```python
from build123d import *

# Parameters (mm, degrees)
BASE_FLANGE1_DEPTH           = 3.175
SKETCH7_R                    = 2.15
CUT_EXTRUDE1_DEPTH           = 10
CUT_EXTRUDE2_DEPTH           = 10
SKETCHED_START               = 19.282254495
SKETCHED_BEND9_OUTLINE_W     = 16.753945323
SKETCHED_BEND9_OUTLINE_H     = 3.175
SKETCHED_BEND9_OUTLINE_W_2   = 24.844698194
SKETCHED_BEND9_OUTLINE_W_3   = 16.78397474
SKETCHED_BEND9_DEPTH         = 24.098637012
SKETCHED_START_2             = 19.005571507
SKETCHED_BEND9_2_OUTLINE_W   = 21.444377118
SKETCHED_BEND9_2_OUTLINE_H   = 3.175
SKETCHED_BEND9_2_DEPTH       = 0.294970988
SKETCHED_START_3             = 13.602941495
SKETCHED_BEND9_3_OUTLINE_R   = 2.15
SKETCHED_BEND9_3_DEPTH       = 6.35
SKETCHED_START_4             = 14.505297696
SKETCHED_BEND9_4_OUTLINE_W   = 1.51683744
SKETCHED_BEND9_4_OUTLINE_H   = 3.175
SKETCHED_BEND9_4_OUTLINE_W_2 = 1.700160538
SKETCHED_BEND9_4_OUTLINE_W_3 = 1.362827281
SKETCHED_BEND9_4_DEPTH       = 0.415197651
SKETCHED_START_5             = 17.361749674
SKETCHED_BEND9_5_DEPTH       = 85
SKETCHED_START_6             = 70.675958021
SKETCHED_BEND9_6_DEPTH       = 16.44868377
SKETCHED_START_7             = 32.782897133
SKETCHED_BEND9_7_DEPTH       = 16.44868377
SKETCHED_START_8             = 49.231580903
SKETCHED_BEND9_8_DEPTH       = 21.444377118


with BuildPart() as part:
    # Base-Flange1: sheet metal written as solids
    # Sketch2 → Base-Flange1 (new body)
    with BuildSketch(Plane(origin=(0, 0, 0), x_dir=(1, 0, 0), z_dir=(0, 1, 0))):
        Polygon((17.361749674, -43.380891507), (102.361749674, -43.380891507), (102.361749674, -20.784622302), (102.361749674, -13.602941495), (102.361749674, 38.619108493), (17.361749674, 38.619108493), align=None)
    extrude(amount=-BASE_FLANGE1_DEPTH)

    # Sketch7 → Cut-Extrude1 (cut)
    with BuildSketch(Plane(origin=(0, 0, 0), x_dir=(1, 0, 0), z_dir=(0, 1, 0))):
        with Locations(Location((54.586454374, -10.030408526, 0), (0, 0, 270))):
            Circle(SKETCH7_R)
        with Locations(Location((93.192772434, -10.030408526, 0), (0, 0, 270))):
            Circle(SKETCH7_R)
        with Locations(Location((93.192772434, 29.969592019, 0), (0, 0, 270))):
            Circle(SKETCH7_R)
        with Locations(Location((54.586454374, 29.969592019, 0), (0, 0, 270))):
            Circle(SKETCH7_R)
        with Locations(Location((94.016482215, -32.082756904, 0), (0, 0, 270))):
            Circle(SKETCH7_R)
        with Locations(Location((59.861749674, -32.082756904, 0), (0, 0, 270))):
            Circle(SKETCH7_R)
        with Locations(Location((25.707017133, -32.082756904, 0), (0, 0, 270))):
            Circle(SKETCH7_R)
    extrude(amount=-CUT_EXTRUDE1_DEPTH, mode=Mode.SUBTRACT)

    # Sketch8 → Cut-Extrude2 (cut)
    with BuildSketch(Plane(origin=(0, 0, 0), x_dir=(1, 0, 0), z_dir=(0, 1, 0))):
        Polygon((85.607804351, -43.380891507), (72.376118559, -43.380891507), (72.376118559, -14.920495347), (70.675958021, -14.920495347), (70.675958021, -12.791720969), (73.98738483, -12.791720969), (73.98738483, -13.602941495), (83.813214982, -13.602941495), (83.813214982, -12.791720969), (87.124641791, -12.791720969), (87.124641791, -14.920495347), (85.607804351, -14.920495347), align=None)
        Polygon((47.531420365, -43.380891507), (34.145724414, -43.380891507), (34.145724414, -14.920495347), (32.782897133, -14.920495347), (32.782897133, -12.791720969), (36.094323942, -12.791720969), (36.094323942, -13.602941495), (45.920154094, -13.602941495), (45.920154094, -12.791720969), (49.231580903, -12.791720969), (49.231580903, -14.920495347), (47.531420365, -14.920495347), align=None)
    extrude(amount=-CUT_EXTRUDE2_DEPTH, mode=Mode.SUBTRACT)

    # Sketched Bend9: read off the stored shape, not the designer's step
    # Sketched Bend9 outline → Sketched Bend9 (cut)
    with BuildSketch(Plane.XY.offset(SKETCHED_START)):
        with Locations((93.984777013, -1.5875)):
            Rectangle(SKETCHED_BEND9_OUTLINE_W, SKETCHED_BEND9_OUTLINE_H)
        with Locations((59.953769462, -1.5875)):
            Rectangle(SKETCHED_BEND9_OUTLINE_W_2, SKETCHED_BEND9_OUTLINE_H)
        with Locations((25.753737044, -1.5875)):
            Rectangle(SKETCHED_BEND9_OUTLINE_W_3, SKETCHED_BEND9_OUTLINE_H)
    extrude(amount=SKETCHED_BEND9_DEPTH, mode=Mode.SUBTRACT)

    # Sketched Bend9 2 outline → Sketched Bend9 2 (cut)
    with BuildSketch(Plane.XY.offset(SKETCHED_START_2)):
        with Locations((59.953769462, -1.5875)):
            Rectangle(SKETCHED_BEND9_2_OUTLINE_W, SKETCHED_BEND9_2_OUTLINE_H)
    extrude(amount=SKETCHED_BEND9_2_DEPTH, mode=Mode.SUBTRACT)

    # Sketched Bend9 3 outline → Sketched Bend9 3 (add)
    # profile 1 of 3: a face of its own
    with BuildSketch(Plane.XY.offset(SKETCHED_START_3)):
        Polygon((85.607804351, -28.946269205), (102.361749674, -28.946269205), (102.361749674, -3.175), (87.124641791, -3.175), (85.607804351, -3.175), align=None)
        with Locations((94.016482215, -17.648134603)):
            Circle(SKETCHED_BEND9_3_OUTLINE_R, mode=Mode.SUBTRACT)
    # profile 2 of 3: a face of its own
    with BuildSketch(Plane.XY.offset(SKETCHED_START_3)):
        Polygon((72.376118559, -28.946269205), (72.376118559, -3.175), (70.675958021, -3.175), (49.231580903, -3.175), (47.531420365, -3.175), (47.531420365, -28.946269205), align=None)
        with Locations((59.861749674, -17.648134603)):
            Circle(SKETCHED_BEND9_3_OUTLINE_R, mode=Mode.SUBTRACT)
    # profile 3 of 3: a face of its own
    with BuildSketch(Plane.XY.offset(SKETCHED_START_3)):
        Polygon((34.145724414, -28.946269205), (34.145724414, -3.175), (32.782897133, -3.175), (17.361749674, -3.175), (17.361749674, -28.946269205), align=None)
        with Locations((25.707017133, -17.648134603)):
            Circle(SKETCHED_BEND9_3_OUTLINE_R, mode=Mode.SUBTRACT)
    extrude(amount=SKETCHED_BEND9_3_DEPTH)

    # Sketched Bend9 4 outline → Sketched Bend9 4 (add)
    with BuildSketch(Plane.XY.offset(SKETCHED_START_4)):
        with Locations((86.366223071, -1.5875)):
            Rectangle(SKETCHED_BEND9_4_OUTLINE_W, SKETCHED_BEND9_4_OUTLINE_H)
        with Locations((71.52603829, -1.5875)):
            Rectangle(SKETCHED_BEND9_4_OUTLINE_W_2, SKETCHED_BEND9_4_OUTLINE_H)
        with Locations((48.381500634, -1.5875)):
            Rectangle(SKETCHED_BEND9_4_OUTLINE_W_2, SKETCHED_BEND9_4_OUTLINE_H)
        with Locations((33.464310774, -1.5875)):
            Rectangle(SKETCHED_BEND9_4_OUTLINE_W_3, SKETCHED_BEND9_4_OUTLINE_H)
    extrude(amount=SKETCHED_BEND9_4_DEPTH)

    # Sketched Bend9 5 outline → Sketched Bend9 5 (cut)
    with BuildSketch(Plane.YZ.offset(SKETCHED_START_5)):
        with BuildLine():
            ThreePointArc((-3.175, 13.602941495), (-4.10493597, 15.848005525), (-6.35, 16.777941495))
            Line((-6.35, 16.777941495), (-28.946269205, 16.777941495))
            Line((-28.946269205, 16.777941495), (-28.946269205, 13.602941495))
            Line((-28.946269205, 13.602941495), (-3.175, 13.602941495))
        make_face()
        with BuildLine():
            Line((0, 13.602941495), (0, 19.282254495))
            Line((0, 19.282254495), (-3.175, 19.282254495))
            Line((-3.175, 19.282254495), (-3.175, 19.952941495))
            Line((-3.175, 19.952941495), (-6.35, 19.952941495))
            ThreePointArc((-6.35, 19.952941495), (-1.859871939, 18.093069556), (0, 13.602941495))
        make_face()
    extrude(amount=SKETCHED_BEND9_5_DEPTH, mode=Mode.SUBTRACT)

    # Sketched Bend9 6 outline → Sketched Bend9 6 (cut)
    with BuildSketch(Plane.YZ.offset(SKETCHED_START_6)):
        with BuildLine():
            Line((-0.261854704, 15.407653897), (-3.305927352, 14.505297696))
            ThreePointArc((-3.305927352, 14.505297696), (-3.20790232, 14.058844085), (-3.175, 13.602941495))
            Line((-3.175, 13.602941495), (-3.175, 14.505297696))
            Line((-3.175, 14.505297696), (-0.064440893, 14.505297696))
            ThreePointArc((-0.064440893, 14.505297696), (-0.146718462, 14.96007014), (-0.261854704, 15.407653897))
        make_face()
    extrude(amount=SKETCHED_BEND9_6_DEPTH, mode=Mode.SUBTRACT)

    # Sketched Bend9 7 outline → Sketched Bend9 7 (cut)
    with BuildSketch(Plane.YZ.offset(SKETCHED_START_7)):
        with BuildLine():
            Line((-0.261854704, 15.407653897), (-3.305927352, 14.505297696))
            ThreePointArc((-3.305927352, 14.505297696), (-3.20790232, 14.058844085), (-3.175, 13.602941495))
            Line((-3.175, 13.602941495), (-3.175, 14.505297696))
            Line((-3.175, 14.505297696), (-0.064440893, 14.505297696))
            ThreePointArc((-0.064440893, 14.505297696), (-0.146718462, 14.96007014), (-0.261854704, 15.407653897))
        make_face()
    extrude(amount=SKETCHED_BEND9_7_DEPTH, mode=Mode.SUBTRACT)

    # Sketched Bend9 8 outline → Sketched Bend9 8 (add)
    with BuildSketch(Plane.YZ.offset(SKETCHED_START_8)):
        with BuildLine():
            Line((-3.175, 19.005571507), (-3.013221769, 19.005571507))
            ThreePointArc((-3.013221769, 19.005571507), (-3.093752415, 19.054487301), (-3.175, 19.10220281))
            Line((-3.175, 19.10220281), (-3.175, 19.005571507))
        make_face()
    extrude(amount=SKETCHED_BEND9_8_DEPTH)


solid = part.part
```
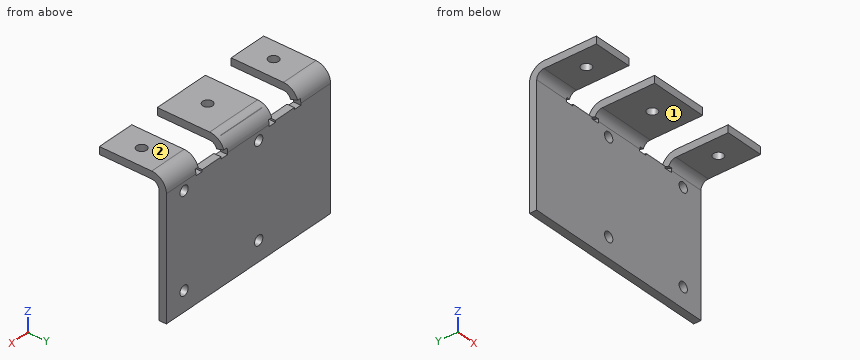
Design review of the part built by this model. Coordinates are the model's own, in mm. Face numbers are marked on the shaded views. A direction names the side the tool comes from. Coordinates: 2 decimals unless noted, no trailing zeros. Loops run counter-clockwise (first coordinate to the right, second up) from the corner with the lowest first, then second, coordinate; pieces in that order, holes last. Notation, with made-up numbers: (57, 13) -> (112, 13) arc R14 cw to (112, 27) -> close; hole circle Ø6 at (-33.75, 16.25). An arc over 180 degrees is marked (long way). Answer as a JSON object with one key per item and string values.
Q1. Take a section at A-A on y = -9.5. Give the boundary of the cut face in (x, z), plus the area to 3 significant figures.
Answer block:
{"outline": "(17.36, 16.78) -> (34.15, 16.78) -> (34.15, 19.95) -> (17.36, 19.95) -> close; (47.53, 16.78) -> (72.38, 16.78) -> (72.38, 19.95) -> (47.53, 19.95) -> close; (85.61, 16.78) -> (102.36, 16.78) -> (102.36, 19.95) -> (85.61, 19.95) -> close", "area": "185 mm^2"}
Q2. Take a section at B-B on x = 63.5. Give the boundary of the cut face in (y, z) (3 decimals).
Answer block:
{"outline": "(-28.946, 16.778) -> (-6.35, 16.778) arc R3.175 cw to (-3.175, 13.603) -> (-3.175, -38.619) -> (0, -38.619) -> (0, 13.603) arc R6.35 ccw to (-6.35, 19.953) -> (-28.946, 19.953) -> close"}
Q3. To check wall thickness, follow L1, parallel to Z at x = 54.5, y = -10.75; L2, parallel to Y at x = 94.5, z = 7.5 (3 decimals); L3, parallel to Z at x = 81, y = -1.5. State the ranges of each line that lie inside material, in increasing order.
Answer block:
{"L1": "z = 16.78 to 19.95", "L2": "y = -3.175 to 0", "L3": "z = -38.62 to 13.6"}
Q4. Tool access review of the marked faces 1 and 2: name each direction out of +Z, -Z, +X, -X, +Y, -Y from which nothing blocks a thin tool from reaching the whole face with its end or side.
Answer block:
{"face 1": "-Z, +X, -X, -Y", "face 2": "+Z, +X, -X, +Y, -Y"}
Q5. Take a section at C-C on z = -29.5. Give the boundary of the cut face in (x, y) (3 decimals).
Answer block:
{"outline": "(17.362, -3.175) -> (52.488, -3.175) -> (52.488, 0) -> (17.362, 0) -> close; (56.685, -3.175) -> (91.095, -3.175) -> (91.095, 0) -> (56.685, 0) -> close; (95.291, -3.175) -> (102.362, -3.175) -> (102.362, 0) -> (95.291, 0) -> close"}
Q6. Take a section at D-D on z = -11. Give the boundary of the cut face in (x, y) (3 decimals).
Answer block:
{"outline": "(17.362, -3.175) -> (102.362, -3.175) -> (102.362, 0) -> (17.362, 0) -> close"}
Q7. Clearance check with flat-ended pins moving along their axes: pin 1 Ø5.5 at (x, y) = (59.86, -17.65) entering from -Z; pin 2 Ø5 at (x, z) = (93.19, 10.03) entering from -Y (3 decimals). State where each tip first meets the part, or that it passes through.
Answer block:
{"pin 1": "stops at z = 16.78", "pin 2": "stops at y = -3.175"}
